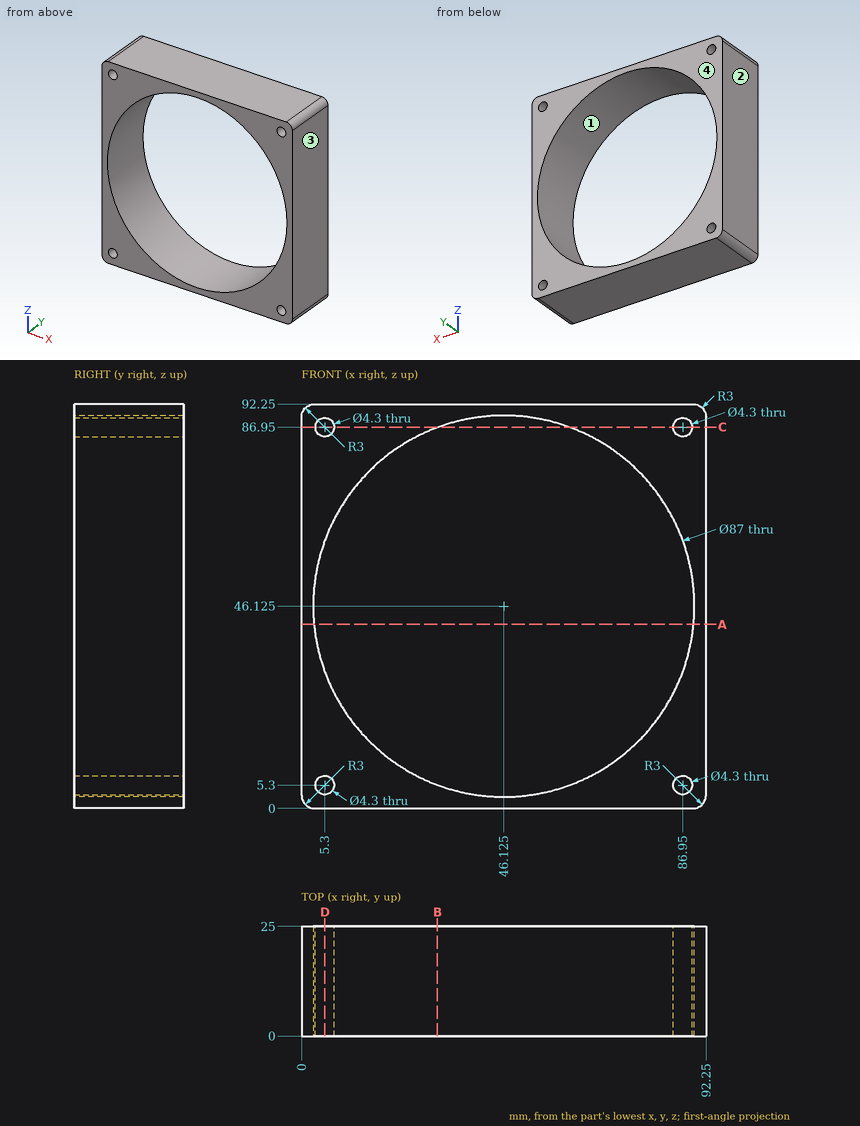
Study the drawing (mm; zero at the part's minimum x, y, z) and answer. Round coordinates to 2 decimals unless told otherwise and drop trailing zeros. Loops run counter-clockwise (first coordinate to the right, second up) from the corner with the lowest first, then second, coordinate; pieces in that order, holes last. Notation, with made-up numbers: (-7.75, -20) -> (7.25, -20) arc R38 ccw to (7.25, 18) -> close; hole circle Ø5 at (82, -7.5). An arc over 180 degrees is marked (long way). One line per item, written item: value.
1) A cutting plane is placed at A-A (z = 42). Determine the outline of the cut face in (x, y).
Answer list:
outline: (0, 0) -> (2.82, 0) -> (2.82, 25) -> (0, 25) -> close; (89.43, 0) -> (92.25, 0) -> (92.25, 25) -> (89.43, 25) -> close
2) A cutting plane is placed at B-B (x = 31). Determine the outline of the cut face in (y, z), and give its area (3 significant figures).
Answer list:
outline: (0, 0) -> (25, 0) -> (25, 5.34) -> (0, 5.34) -> close; (0, 86.91) -> (25, 86.91) -> (25, 92.25) -> (0, 92.25) -> close
area: 267 mm²
3) A cutting plane is placed at C-C (z = 86.95). Determine the outline of the cut face in (x, y), and give its area (3 significant figures).
Answer list:
outline: (0, 0) -> (3.15, 0) -> (3.15, 25) -> (0, 25) -> close; (7.45, 0) -> (31.11, 0) -> (31.11, 25) -> (7.45, 25) -> close; (61.14, 0) -> (84.8, 0) -> (84.8, 25) -> (61.14, 25) -> close; (89.1, 0) -> (92.25, 0) -> (92.25, 25) -> (89.1, 25) -> close
area: 1,340 mm²
4) Consider L1, parallel to Z at x = 52, y = 12; L2, parallel to X at y = 3.5, z = 45; L3, parallel to X at y = 15, z = 72.5. Determine where each line is inside the solid, lowest interval first. Write a range as [from, to].
Answer list:
L1: z = [0, 3.02], [89.23, 92.25]
L2: x = [0, 2.64], [89.61, 92.25]
L3: x = [0, 11.53], [80.72, 92.25]
5) A cutting plane is placed at D-D (x = 5.3). Determine the outline of the cut face in (y, z), and give its area (3 significant figures).
Answer list:
outline: (0, 0) -> (25, 0) -> (25, 3.15) -> (0, 3.15) -> close; (0, 7.45) -> (25, 7.45) -> (25, 31.11) -> (0, 31.11) -> close; (0, 61.14) -> (25, 61.14) -> (25, 84.8) -> (0, 84.8) -> close; (0, 89.1) -> (25, 89.1) -> (25, 92.25) -> (0, 92.25) -> close
area: 1,340 mm²
6) The mould has two halves that part along X. Classify the marked faces 1, 2, 3 and 4: pulls with the +X half, pulls with the -X half, needs draft (parallel to the pull), parting line crosses it, or undercut.
Answer list:
face 1: undercut
face 2: pulls with the -X half
face 3: pulls with the +X half
face 4: needs draft
